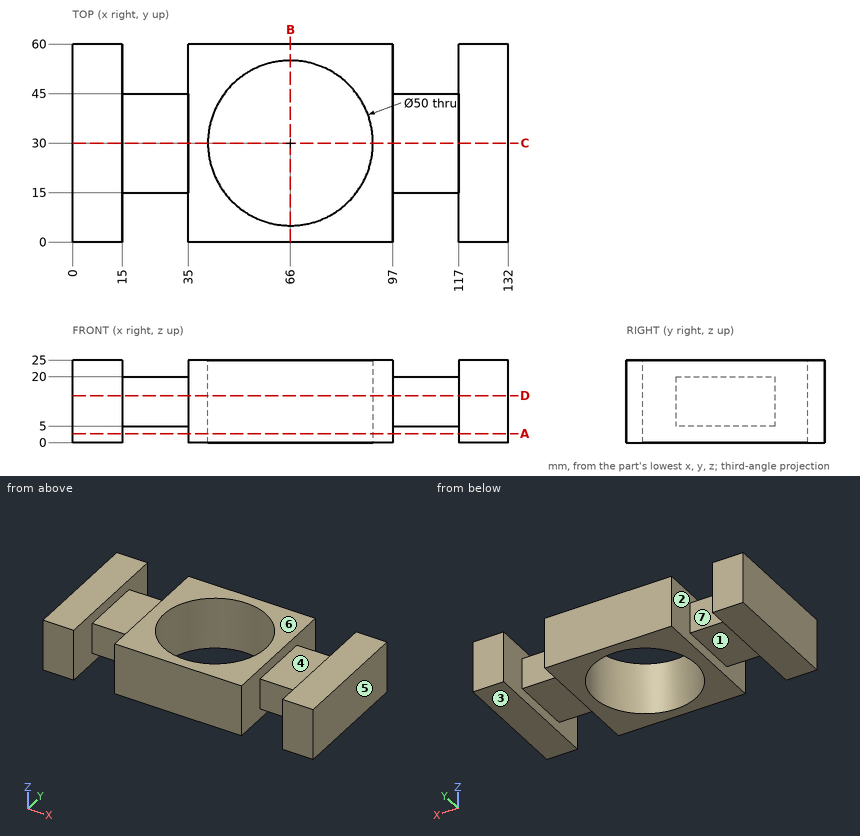
Job drawing, mm, ordinate dimensions from the low corner. One solid piece. A direction names the side the tool comes from. Round coordinates to 2 decimals unless told otherwise and drop trailing zeros. Loops run counter-clockwise (first coordinate to the right, second up) from the corner with the lowest first, then second, coordinate; pieces in that order, holes last.
(1) Cut at B-B (x = 66). Give the cut face in (y, z), plus the area to 3 significant figures.
(2) Drop flat-ended pins along their axis: pin 1 (4.5 mm diameter, centred on x = 103.5, z = 14.5, fed in from -Y); pin 2 (4 mm diameter, centred on x = 19, z = 6, fed in from +Y); pin 3 (6 mm diameter, centred on x = 27, y = 36.5, fed in from -Z). Give the stop position or say it passes through.
(3) Which spindle directions (+Z, -Z, +X, -X, +Y, -Y) get a long thin tool onto all of the face, cutting with end or side? Do the marked faces 1, 2 and 3. Say none if no direction does.
(4) Two-plate mould, pull along X, no slides. Class the marked faces 4, 5, 6 and 7: +X half, -X half, draft (parallel to the pull), parting line (faces both ways), or undercut.
(5) Cut at D-D (z = 14.25). Give the cut face in (x, y), plus the area to 3 significant figures.
(6) Cut at C-C (y = 30). Give the cut face in (x, z).
(7) Wall check: line 1 along Y through (x, z) = (66, 19.75); line 2 along X through (y, z) = (30.5, 1.5) (3 decimals); line 3 along X through (y, z) = (53, 16.25). Give the ranges that are in metal, low to high.
(8) Cut at A-A (z = 2.75). Give the cut face in (x, y), plus the area to 3 significant figures.
Findings below:
1. outline: (0, 0) - (5, 0) - (5, 25) - (0, 25) - close; (55, 0) - (60, 0) - (60, 25) - (55, 25) - close
1. area: 250 mm2
2. pin 1: stops at y = 15
2. pin 2: stops at y = 45
2. pin 3: stops at z = 5
3. face 1: -Z, +Y, -Y
3. face 2: none
3. face 3: -Z, +X, -X, +Y, -Y
4. face 4: undercut
4. face 5: +X half
4. face 6: draft
4. face 7: undercut
5. outline: (0, 0) - (15, 0) - (15, 15) - (35, 15) - (35, 0) - (97, 0) - (97, 15) - (117, 15) - (117, 0) - (132, 0) - (132, 60) - (117, 60) - (117, 45) - (97, 45) - (97, 60) - (35, 60) - (35, 45) - (15, 45) - (15, 60) - (0, 60) - close; hole circle Ø50 at (66, 30)
5. area: 4,760 mm2
6. outline: (0, 0) - (15, 0) - (15, 5) - (35, 5) - (35, 0) - (41, 0) - (41, 25) - (35, 25) - (35, 20) - (15, 20) - (15, 25) - (0, 25) - close; (91, 0) - (97, 0) - (97, 5) - (117, 5) - (117, 0) - (132, 0) - (132, 25) - (117, 25) - (117, 20) - (97, 20) - (97, 25) - (91, 25) - close
7. line 1: y = 0 to 5, 55 to 60
7. line 2: x = 0 to 15, 35 to 41.005, 90.995 to 97, 117 to 132
7. line 3: x = 0 to 15, 35 to 56.2, 75.8 to 97, 117 to 132
8. outline: (0, 0) - (15, 0) - (15, 60) - (0, 60) - close; (35, 0) - (97, 0) - (97, 60) - (35, 60) - close; (117, 0) - (132, 0) - (132, 60) - (117, 60) - close; hole circle Ø50 at (66, 30)
8. area: 3,560 mm2
